For this review, take the finished solid that the model builds, in its own axes (mm). Face numbers are marked on the shaded views. A direction names the side the tool comes from. Coordinates: 2 decimals unless noted, no trailing zeros. Write each loop counter-clockwise with the first axis right and the second up, starting at its lowest first coordinate (ties: lowest second). Pieces come first, ordered by that corner, then holes.
```python
from build123d import *

# Parameters (mm, degrees)
F0_W     = 50.8
F0_H     = 25.4
F1_DEPTH = 25.4
F2_R     = 3.81
F3_DEPTH = 63.5
F6_SIZE  = 5.08


with BuildPart() as f1:
    # F0 (on Top) → F1 (new body)
    with BuildSketch(Plane.XY):
        with Locations((0, -1.165138)):
            Rectangle(F0_W, F0_H)
    extrude(amount=F1_DEPTH)

    # F2 (on face) → F3 (join)
    with BuildSketch(Plane.XY.offset(25.4)):
        Circle(F2_R)
    extrude(amount=F3_DEPTH)

    # F4 (on face) → F5 (revolve)
    with BuildSketch(Plane.XY.offset(88.9)):
        with BuildLine():
            Line((0, 3.81), (0, -3.81))
            ThreePointArc((0, -3.81), (2.694077, -2.694077), (3.81, 0))
            ThreePointArc((3.81, 0), (2.694077, 2.694077), (0, 3.81))
        make_face()
    revolve(axis=Axis((0, 0, 88.9), (0, -1, 0)))

    # F6
    f6_edges = [f1.edges().sort_by_distance(p)[0] for p in [
        (-25.4, 11.534862, 12.7),
        (-25.4, -1.165138, 25.4),
        (25.4, -1.165138, 25.4),
        (25.4, 11.534862, 12.7),
        (25.4, -1.165138, 0),
        (25.4, -13.865138, 12.7),
        (-25.4, -13.865138, 12.7),
        (-25.4, -1.165138, 0),
    ]]
    chamfer(f6_edges, length=F6_SIZE)


solid = f1.part
```
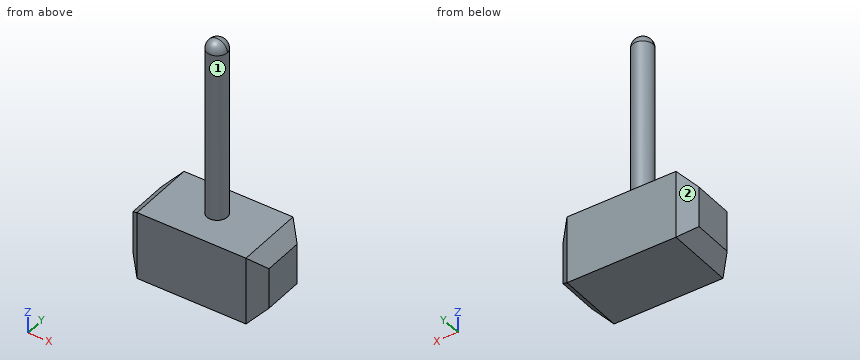
Q1. Clearance check with flat-ended pins moving along their axes: pin 1 Ø1 at (x, y) = (-8.5, -8) entering from +Z; pin 2 Ø12 at (y, z) = (-3, 65.5) entering from -X; pin 3 Ø1 at (y, z) = (-3, 58.5) entering from -X; pin 4 Ø6 at (x, z) = (9.5, 55) entering from -Y. State where each tip first meets the part, or that it passes through.
Ans:
pin 1: stops at z = 25.4
pin 2: stops at x = -3.81
pin 3: stops at x = -2.88
pin 4: passes through
Q2. Add section B-B (y = -10). State the section outline as (x, z) points.
Ans:
outline: (-24.19, 3.87) - (-20.32, 0) - (20.32, 0) - (24.19, 3.87) - (24.19, 21.53) - (20.32, 25.4) - (-20.32, 25.4) - (-24.19, 21.53) - close
Q3. For probe 1 along Z at (x, y) = (0, 4.5); probe 2 along X at (y, z) = (-1, 4); probe 3 along X at (y, z) = (3.5, 86), list the stretches that pass through material, from the lowest coordinate up.
Ans:
probe 1: z = 0 to 25.4
probe 2: x = -24.32 to 24.32
probe 3: x = -1.51 to 1.51
Q4. Tool access review of the marked faces 1 and 2: name each direction out of +Z, -Z, +X, -X, +Y, -Y from which nothing blocks a thin tool from reaching the whole face with its end or side.
Ans:
face 1: +Z
face 2: +Z, -Z, -X, +Y
Q5. Add section C-C (z = 49.5). State the section outline as (x, y) points, then the cut area to 3 significant figures.
Ans:
outline: circle Ø7.62 at (0, 0)
area: 45.6 mm2
Q6. Add section A-A (z = 11). State the section outline as (x, y) points, then the cut area to 3 significant figures.
Ans:
outline: (-25.4, -8.79) - (-20.32, -13.87) - (20.32, -13.87) - (25.4, -8.79) - (25.4, 6.45) - (20.32, 11.53) - (-20.32, 11.53) - (-25.4, 6.45) - close
area: 1,240 mm2
